from build123d import *

# Parameters (mm, degrees)
EXTRUDE_1_DEPTH      = 45
EXTRUDE_1_DEPTH_BACK = 45
CUT_EXTRUDE_1_DEPTH  = 61
SKETCH_4_R           = 2.5
CUT_EXTRUDE_2_DEPTH  = 61
SKETCH_5_R           = 4
CUT_EXTRUDE_3_DEPTH  = 50


with BuildPart() as part:
    # Sketch 1 → Extrude 1 (new body, two sides)
    with BuildSketch(Plane.XY) as extrude_1_sk:
        Polygon((30, -4.983496438), (-30, -4.983496438), (-30, 48.016503562), (-28, 48.016503562), (-28, -2.983496438), (28, -2.983496438), (28, 48.016503562), (30, 48.016503562), align=None)
    extrude(amount=EXTRUDE_1_DEPTH)
    extrude(extrude_1_sk.sketch, amount=-EXTRUDE_1_DEPTH_BACK)

    # Sketch 3 → Cut-Extrude 1 (cut, through all)
    with BuildSketch(Plane(origin=(30, 0, 0), x_dir=(0, 0, -1), z_dir=(1, 0, 0))):
        with BuildLine():
            Line((-45, 48.016503562), (-45, 3.016503562))
            ThreePointArc((-45, 3.016503562), (-31.819805121, 34.836308748), (9.2e-08, 48.016503562))
            Line((9.2e-08, 48.016503562), (-45, 48.016503562))
        make_face()
        with BuildLine():
            Line((45, 48.016503562), (9.2e-08, 48.016503562))
            ThreePointArc((9.2e-08, 48.016503562), (31.819805186, 34.836308683), (45, 3.016503562))
            Line((45, 3.016503562), (45, 48.016503562))
        make_face()
    extrude(amount=-CUT_EXTRUDE_1_DEPTH, mode=Mode.SUBTRACT)

    # Sketch 4 → Cut-Extrude 2 (cut, through all)
    with BuildSketch(Plane.ZY.offset(30)):
        with Locations((0, 26.516503562)):
            Circle(SKETCH_4_R)
    extrude(amount=-CUT_EXTRUDE_2_DEPTH, mode=Mode.SUBTRACT)

    # Sketch 5 → Cut-Extrude 3 (cut)
    with BuildSketch(Plane.XZ.offset(4.983496438)):
        Circle(SKETCH_5_R)
    extrude(amount=-CUT_EXTRUDE_3_DEPTH, mode=Mode.SUBTRACT)


solid = part.part
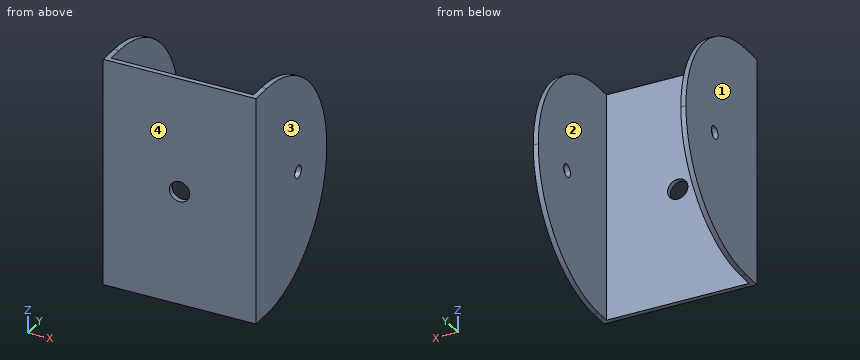
Can you work these out from the model? Positions are in its coordinate system, mm. Face numbers are marked on the shaded views. Round coordinates to 2 decimals unless told otherwise and drop trailing zeros. Write each loop counter-clockwise with the first axis right and the second up, starting at its lowest first coordinate (ties: lowest second). Pieces come first, ordered by that corner, then holes. Notation, with made-up numbers: (32.5, 11.5) -> (39.5, 11.5) arc R27 ccw to (39.5, 37.5) -> close; hole circle Ø11 at (45, 23). An arc over 180 degrees is marked (long way). One line per question, with ' | ' between items. Start each with the question number.
1) I'm going to push flat-ended pins straight in: P1, Ø6, axis at y = 26.52, z = 0, coming from the -X side; P2, Ø1, axis at x = 12.5, z = 24.5, coming from the +Y side. Where does each tip first touch, or does it pass through?
2) I need wall thicknesses on line 1 (Y direction, x = -29.6, z = 0); line 2 (X direction, y = 4, z = 17); line 3 (Z direction, x = 0, y = -3.5). Which ranges of each line are inside material? Lowest first, please. Write a range as [from, to].
3) If we mould it in two halves opening along X, with no side actions, what happens to the marked faces 1, 2, 3 and 4? For each: released by +X, released by -X, zero draft, split by the parting line, or undercut.
4) Suppose I cut it at A-A on x = 0. Write out the boundary of the cut face in (y, z), then the cut area to 3 significant figures.
5) Suppose I cut it at C-C on z = 6. Write out the boundary of the cut face in (x, y).
6) Suppose I cut it at D-D on x = 12.5. Write out the boundary of the cut face in (y, z).
7) Suppose I cut it at B-B on y = 1.5. Write out the boundary of the cut face in (x, z).
Return value:
1) P1: stops at x = -30 | P2: stops at y = -2.98
2) line 1: y = [-4.98, 24.02], [29.02, 48.02] | line 2: x = [-30, -28], [28, 30] | line 3: z = [-45, -4], [4, 45]
3) face 1: released by -X | face 2: undercut | face 3: released by +X | face 4: zero draft
4) outline: (-4.98, -45) -> (-2.98, -45) -> (-2.98, -4) -> (-4.98, -4) -> close; (-4.98, 4) -> (-2.98, 4) -> (-2.98, 45) -> (-4.98, 45) -> close | area: 164 mm2
5) outline: (-30, -4.98) -> (30, -4.98) -> (30, 47.61) -> (28, 47.61) -> (28, -2.98) -> (-28, -2.98) -> (-28, 47.61) -> (-30, 47.61) -> close
6) outline: (-4.98, -45) -> (-2.98, -45) -> (-2.98, 45) -> (-4.98, 45) -> close
7) outline: (-30, -45) -> (-28, -45) -> (-28, 45) -> (-30, 45) -> close; (28, -45) -> (30, -45) -> (30, 45) -> (28, 45) -> close
